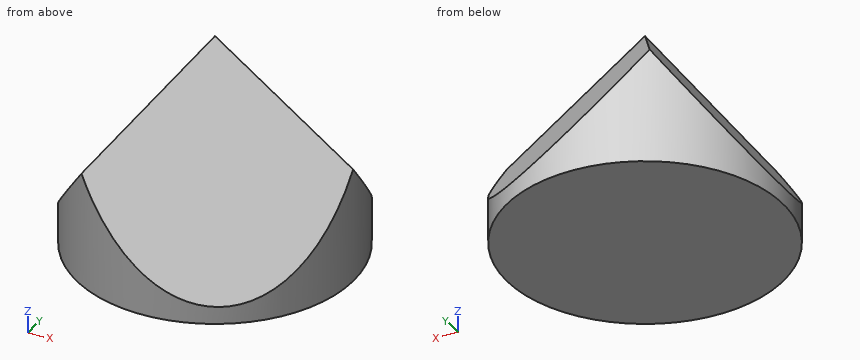
```python
from build123d import *

# Parameters (mm, degrees)
SKETCH_1_R          = 31.1
EXTRUDE_1_DEPTH     = 47.9
CUT_EXTRUDE_1_DEPTH = 39.5
CUT_EXTRUDE_2_DEPTH = 62
CUT_EXTRUDE_3_DEPTH = 53.5


with BuildPart() as part:
    # 草图1 → 凸台-拉伸1 (new body)
    with BuildSketch(Plane.XY):
        Circle(SKETCH_1_R)
    extrude(amount=EXTRUDE_1_DEPTH)

    # 草图2 → 切除-拉伸1 (cut, symmetric)
    with BuildSketch(Plane(origin=(0, 0, 0), x_dir=(1, 0, 0), z_dir=(0, 1, 0))):
        Polygon((0, -47.9), (-40.690324156, 9.632856926), (-40.690324156, -56.656954578), (0, -56.656954578), align=None)
    extrude(amount=CUT_EXTRUDE_1_DEPTH, both=True, mode=Mode.SUBTRACT)

    # 草图4 → 切除-拉伸2 (cut, symmetric)
    with BuildSketch(Plane(origin=(0, 0, 0), x_dir=(0.5, 0.866025404, 0), z_dir=(0.866025404, -0.5, 0))):
        Polygon((0, 47.9), (100.699346514, -94.480804669), (100.699346514, 79.089205692), (0, 79.089205692), align=None)
    extrude(amount=CUT_EXTRUDE_2_DEPTH, both=True, mode=Mode.SUBTRACT)

    # 草图5 → 切除-拉伸3 (cut, symmetric)
    with BuildSketch(Plane(origin=(0, 0, 0), x_dir=(0.5, -0.866025404, 0), z_dir=(-0.866025404, -0.5, 0))):
        Polygon((0, 47.9), (45.690289371, -16.702406981), (45.690289371, 62.081252558), (2.684670532, 62.081252558), align=None)
    extrude(amount=CUT_EXTRUDE_3_DEPTH, both=True, mode=Mode.SUBTRACT)


solid = part.part
```
Geometry: final body of the model. Coordinates: model frame, mm. Coordinates: 2 decimals unless noted, no trailing zeros. Loops run counter-clockwise (first coordinate to the right, second up) from the corner with the lowest first, then second, coordinate; pieces in that order, holes last. Notation, with made-up numbers: (13.25, 73.25) -> (18.25, 73.25) arc R18 ccw to (18.25, 108.25) -> close; hole circle Ø6 at (45, 45.25). An arc over 180 degrees is marked (long way). Use a Markdown table: item, result. Add a question column.
(1) Section query A-A, the plane z = 3. Return loops of the section in (x, y), plus the area to 3 significant figures.
(2) Pin query (flat end, axial travel): pin 1 Ø12 at (x, y) = (5, -23.5) entering from +Z; pin 2 Ø5 at (x, z) = (19, 5) entering from -Y; pin 3 Ø10 at (x, z) = (-6, 12.5) entering from +Y. Return the tip coordinate at first contact, or that it passes through.
(3) Line query: line 1 along Y through (x, z) = (15.5, 14); line 2 along Y through (x, z) = (14.5, 15); line 3 along X through (y, z) = (-4, 28.5). Output: solid intervals per line, ascending.
(4) Section query B-B, the plane y = -16.5. Return loops of the section in (x, z), plus the area to 3 significant figures.
(5) Section query D-D, the plane z = 25. Return loops of the section in (x, y), plus the area to 3 significant figures.
(6) Section query C-C, the plane x = 23. Return loops of the section in (y, z), plus the area to 3 significant figures.
Answer:
| question | item | result |
|---|---|---|
| 1 | outline | circle Ø62.2 at (0, 0) |
| 1 | area | 3,040 mm^2 |
| 2 | pin 1 | stops at z = 24.07 |
| 2 | pin 2 | stops at y = -26.22 |
| 2 | pin 3 | stops at y = 31.07 |
| 3 | line 1 | y = -18.74 to 18.74 |
| 3 | line 2 | y = -18.5 to 18.5 |
| 3 | line 3 | x = -13.72 to 20.51 |
| 4 | outline | (-26.36, 0) -> (26.36, 0) -> (26.36, 9.06) -> (-9.53, 34.43) -> (-26.36, 10.63) -> close |
| 4 | area | 1,160 mm^2 |
| 5 | outline | (-16.2, -26.55) arc R31.1 ccw to (-14.89, -27.3) -> (31.09, -0.75) arc R31.1 ccw to (31.09, 0.75) -> (-14.89, 27.3) arc R31.1 ccw to (-16.2, 26.55) -> close |
| 5 | area | 1,360 mm^2 |
| 6 | outline | (-20.93, 0) -> (20.93, 0) -> (20.93, 6.01) -> (0, 31.64) -> (-20.93, 6.01) -> close |
| 6 | area | 788 mm^2 |
